Input: dimensioned drawing with shaded views. Units: mm. Origin: part minimum x, y, z. A direction names the side the tool comes from. Round coordinates to 2 decimals unless told otherwise and drop trailing zeros. Order: outer loops, then holes, each group sorted by start corner. A loop starts at its lowest first (then second) coordinate and runs counter-clockwise, first axis right, second up. Notation, with made-up numbers: (-15.5, 72.25) - (32.5, 72.25) arc R31 ccw to (32.5, 104.25) - close; hole circle Ø5 at (22, -29.75). An arc over 180 degrees is marked (long way). One line per item, written item: value. Start each with the question number.
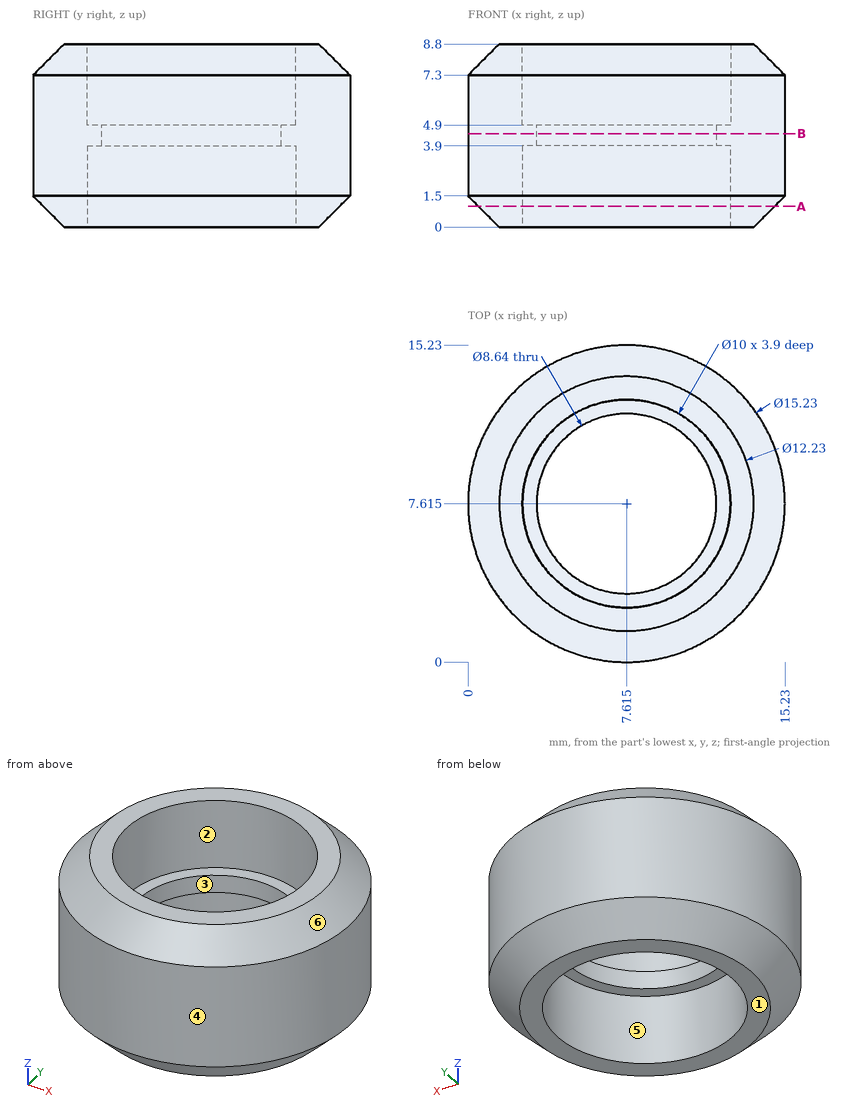
1. Pin query (flat end, axial travel): pin 1 (1 mm diameter, centred on y = 10, z = 6, fed in from -X); pin 2 (4 mm diameter, centred on x = 9.5, y = 9.5, fed in from -Z); pin 3 (1.5 mm diameter, centred on x = 13.5, y = 12, fed in from -Z). Return the tip coordinate at first contact, or that it passes through.
2. Section A-A (z = 1). Return the cut outline in (x, y) (3 decimals), then the cut area to 3 significant figures.
3. Pull-direction query (X, two-part tool) for the marked faces 1, 2, 3 and 4; classes: released by +X, released by -X, zero draft, split by the parting line, or undercut.
4. Line query: line 1 (X direction, y = 7.75, z = 4.5); line 2 (Y direction, x = 11, z = 6.5); line 3 (Y direction, x = 9.25, z = 1.25). Output: solid intervals per line, ascending. Write a range as from..to.
5. Section B-B (z = 4.5). Return the cut outline in (x, y) (3 decimals), then the cut area to 3 significant figures.
6. Set-up query: the marked faces 5 and 6. Return all of +Z, -Z, +X, -X, +Y, -Y with unobstructed straight access to the full face (end or side cutting, diameter ignored); none if empty.
Solved:
1. pin 1: stops at x = 0.24
1. pin 2: stops at z = 3.9
1. pin 3: stops at z = 0.47
2. outline: circle Ø14.23 at (7.615, 7.615); hole circle Ø10 at (7.615, 7.615)
2. area: 80.5 mm²
3. face 1: zero draft
3. face 2: undercut
3. face 3: undercut
3. face 4: split by the parting line
4. line 1: x = 0..3.3, 11.93..15.23
4. line 2: y = 0.79..3.94, 11.29..14.44
4. line 3: y = 0.43..2.89, 12.34..14.8
5. outline: circle Ø15.23 at (7.615, 7.615); hole circle Ø8.64 at (7.615, 7.615)
5. area: 124 mm²
6. face 5: -Z
6. face 6: +Z
